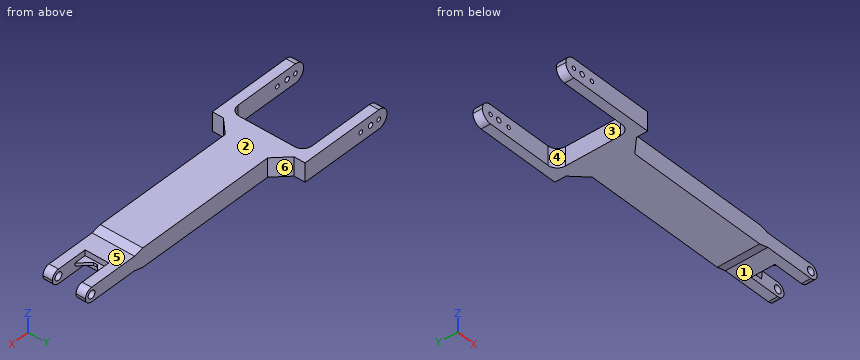
```python
from build123d import *

# Parameters (mm, degrees)
SKETCH_2_W          = 187.5
SKETCH_2_H          = 45.3
EXTRUDE_1_DEPTH     = 10
EXTRUDE_2_DEPTH     = 7.5
CHAMFER_1_SIZE      = 20
CHAMFER_1_SIZE_2    = 5
CHAMFER_2_SIZE      = 5
CHAMFER_2_SIZE_2    = 20
EXTRUDE_3_DEPTH     = 1.5
CHAMFER_3_SIZE      = 3
CUT_EXTRUDE_1_DEPTH = 314.699298692
CUT_EXTRUDE_2_DEPTH = 307.287238552
CHAMFER_4_SIZE      = 15
FILLET_1_R          = 10


with BuildPart() as part:
    # 草图2 → 凸台-拉伸1 (new, symmetric)
    with BuildSketch(Plane.XY):
        with Locations((-103.75, 0)):
            Rectangle(SKETCH_2_W, SKETCH_2_H)
        Polygon((-297.5, 49.5), (-297.5, 39.5), (-207.5, 39.5), (-207.5, -39.5), (-297.5, -39.5), (-297.5, -49.5), (-197.5, -49.5), (-197.5, 49.5), align=None)
    extrude(amount=EXTRUDE_1_DEPTH, both=True)

    # 草图2<3> → 凸台-拉伸2 (add, symmetric)
    with BuildSketch(Plane.XY):
        Polygon((40, -22.65), (40, -12.65), (0, -12.65), (0, 12.65), (40, 12.65), (40, 22.65), (-10, 22.65), (-10, -22.65), align=None)
    extrude(amount=EXTRUDE_2_DEPTH, both=True)

    # 倒角1
    # the kernel refuses this chamfer: 20, 5 mm, written as the material it takes off along each edge
    with BuildSketch(Plane(origin=(-10, -74.592549995, 10), x_dir=(-0.9999563942249224, 0, 0.00933861064031752), z_dir=(0, 1, 0))) as chamfer_1_piece_1_section:
        Polygon((CHAMFER_1_SIZE * 0.999956394225, -CHAMFER_1_SIZE * 0.00933861064032), (-CHAMFER_1_SIZE_2 * 0.00933861064032, -CHAMFER_1_SIZE_2 * 0.999956394225), (0, 0), align=None)
    chamfer_1_piece_1 = extrude(amount=149.185099991, mode=Mode.PRIVATE)
    chamfer_1_piece_1 = split(chamfer_1_piece_1, bisect_by=Plane(origin=(-18.245866107, 0, 7.5), z_dir=(0, 0, 1)), keep=Keep.TOP, mode=Mode.PRIVATE)
    add(chamfer_1_piece_1, mode=Mode.SUBTRACT)

    # 倒角2
    # the kernel refuses this chamfer: 20, 5 mm, written as the material it takes off along each edge
    with BuildSketch(Plane(origin=(-10, -74.592549995, -10), x_dir=(0.14778356633657133, 0, 0.9890197255468893), z_dir=(0, 1, 0))) as chamfer_2_piece_1_section:
        Polygon((CHAMFER_2_SIZE * 0.989019725547, -CHAMFER_2_SIZE * 0.147783566337), (-CHAMFER_2_SIZE_2 * 0.147783566337, -CHAMFER_2_SIZE_2 * 0.989019725547), (0, 0), align=None)
    chamfer_2_piece_1 = extrude(amount=149.185099991, mode=Mode.PRIVATE)
    chamfer_2_piece_1 = split(chamfer_2_piece_1, bisect_by=Plane(origin=(-18.245866107, 0, -7.5), z_dir=(0, 0, -1)), keep=Keep.TOP, mode=Mode.PRIVATE)
    add(chamfer_2_piece_1, mode=Mode.SUBTRACT)

    # 草图2<5> → 凸台-拉伸3 (add, symmetric)
    with BuildSketch(Plane.XY):
        Polygon((12.65, 12.65), (0, 12.65), (0, 0), align=None)
        Polygon((12.65, -12.65), (0, 0), (0, -12.65), align=None)
    extrude(amount=EXTRUDE_3_DEPTH, both=True)

    # 倒角3
    chamfer_3_edges = [part.edges().sort_by_distance(p)[0] for p in [
        (0, 0, 0),
    ]]
    chamfer(chamfer_3_edges, length=CHAMFER_3_SIZE)

    # 草图3 → 切除-拉伸1 (cut, through all)
    with BuildSketch(Plane(origin=(0, 49.5, 0), x_dir=(1, 0, 0), z_dir=(0, 1, 0))):
        with BuildLine():
            ThreePointArc((-297.5, 0), (-294.571067812, 7.071067812), (-287.5, 10))
            Line((-287.5, 10), (-297.5, 10))
            Line((-297.5, 10), (-297.5, 0))
        make_face()
        with BuildLine():
            Line((-297.5, -10), (-287.5, -10))
            ThreePointArc((-287.5, -10), (-294.571067812, -7.071067812), (-297.5, 0))
            Line((-297.5, 0), (-297.5, -10))
        make_face()
        with BuildLine():
            ThreePointArc((-289.65, 0), (-287.5, -2.15), (-285.35, 0))
            Line((-285.35, 0), (-289.65, 0))
        make_face()
        with BuildLine():
            Line((-289.65, 0), (-285.35, 0))
            ThreePointArc((-285.35, 0), (-287.5, 2.15), (-289.65, 0))
        make_face()
        with BuildLine():
            ThreePointArc((-280.15, 0), (-277.5, -2.65), (-274.85, 0))
            Line((-274.85, 0), (-280.15, 0))
        make_face()
        with BuildLine():
            Line((-280.15, 0), (-274.85, 0))
            ThreePointArc((-274.85, 0), (-277.5, 2.65), (-280.15, 0))
        make_face()
        with BuildLine():
            ThreePointArc((-267.65, 0), (-265.5, -2.15), (-263.35, 0))
            Line((-263.35, 0), (-267.65, 0))
        make_face()
        with BuildLine():
            Line((-267.65, 0), (-263.35, 0))
            ThreePointArc((-263.35, 0), (-265.5, 2.15), (-267.65, 0))
        make_face()
    extrude(amount=-CUT_EXTRUDE_1_DEPTH, mode=Mode.SUBTRACT)

    # 草图4 → 切除-拉伸2 (cut, through all)
    with BuildSketch(Plane(origin=(0, 22.65, 0), x_dir=(1, 0, 0), z_dir=(0, 1, 0))):
        with BuildLine():
            ThreePointArc((28.35, 0), (32.5, -4.15), (36.65, 0))
            Line((36.65, 0), (28.35, 0))
        make_face()
        with BuildLine():
            Line((28.35, 0), (36.65, 0))
            ThreePointArc((36.65, 0), (32.5, 4.15), (28.35, 0))
        make_face()
        with BuildLine():
            ThreePointArc((32.5, 7.5), (37.803300859, 5.303300859), (40, 0))
            Line((40, 0), (40, 7.5))
            Line((40, 7.5), (32.5, 7.5))
        make_face()
        with BuildLine():
            Line((40, -7.5), (40, 0))
            ThreePointArc((40, 0), (37.80330088, -5.303300838), (32.500000061, -7.5))
            Line((32.500000061, -7.5), (40, -7.5))
        make_face()
    extrude(amount=-CUT_EXTRUDE_2_DEPTH, mode=Mode.SUBTRACT)

    # 倒角4
    chamfer_4_edges = [part.edges().sort_by_distance(p)[0] for p in [
        (-197.5, -22.65, 0),
        (-197.5, 22.65, 0),
    ]]
    chamfer(chamfer_4_edges, length=CHAMFER_4_SIZE)

    # 圆角1
    fillet_1_edges = [part.edges().sort_by_distance(p)[0] for p in [
        (-207.5, -39.5, 0),
        (-207.5, 39.5, 0),
    ]]
    fillet(fillet_1_edges, radius=FILLET_1_R)


solid = part.part
```
Input: part model. Units: mm. Frame: model coordinates. Face numbers are marked on the shaded views. A direction names the side the tool comes from. Round coordinates to 2 decimals unless told otherwise and drop trailing zeros. Write each loop counter-clockwise with the first axis right and the second up, starting at its lowest first coordinate (ties: lowest second). Pieces come first, ordered by that corner, then holes. Notation, with made-up numbers: M -15,39 L 19,39 A32 cw 19,73 Z; hole C -12,53.5 d1. An arc over 180 degrees is marked long. Write each question's results on one line, items separated by ' | '.
Q1. Line query: line 1 along Z through (x, y) = (32, 16); line 2 along Y through (x, z) = (-230, -2); line 3 along Z through (x, y) = (-287.5, 46.75). Output: solid intervals per line, ascending.
Results:
line 1: z = -7.5 to -4.12, 4.12 to 7.5 | line 2: y = -49.5 to -39.5, 39.5 to 49.5 | line 3: z = -10 to -2.15, 2.15 to 10
Q2. Section query B-B (x = -109). Return loops of the section in (y, z), and give its area (3 significant figures).
Results:
outline: M -22.65,-10 L 22.65,-10 L 22.65,10 L -22.65,10 Z | area: 906 mm^2
Q3. Section query A-A (y = -17). Return loops of the section in (x, z).
Results:
outline: M -207.5,-10 L -30,-10 L -20,-7.5 L 32.5,-7.5 A7.5 ccw 32.5,7.5 L -20,7.5 L -30,10 L -207.5,10 Z; hole C 32.5,0 d8.3
Q4. Access query for the marked faces 1, 2 and 3. Directions: +Z, -Z, +X, -X, +Y, -Y. A direction counts if a zero-diameter tool reaches every point of the face in a straight line with its end or side. Return the directions, or none.
Results:
face 1: -Z, +X, +Y, -Y | face 2: +Z, +X, -X, +Y, -Y | face 3: +Z, -Z, -X
Q5. Pin query (flat end, axial travel): P1, Ø4, axis at y = 26.5, z = -5.5, coming from the -X side; P2, Ø4, axis at x = -287.5, z = 0, coming from the -Y side; P3, Ø12, axis at x = -48.5, z = 2, coming from the -Y side; P4, Ø3.5, axis at y = -45.5, z = -2, coming from the +X side. Return the tip coordinate at first contact, or that it passes through.
Results:
P1: stops at x = -207.5 | P2: passes through | P3: stops at y = -22.65 | P4: stops at x = -197.5
Q6. Draft query along Y for the marked faces 4, 5 and 6. Return one class per face: released by +Y, released by -Y, zero draft, split by the parting line, or undercut.
Results:
face 4: undercut | face 5: zero draft | face 6: released by +Y
Q7. Section query C-C (y = -33). Return loops of the section in (x, z).
Results:
outline: M -208.13,-10 L -192.85,-10 L -192.85,10 L -208.13,10 Z
